from build123d import *

# Parameters (mm, degrees)
CUT_EXTRUDE_1_DEPTH = 4.5
CHAMFER_1_SIZE      = 0.5


with BuildPart() as part:
    # Эскиз1 → Повернуть1 (revolve)
    with BuildSketch(Plane.XY, mode=Mode.PRIVATE) as revolve_1_sk:
        with BuildLine():
            Line((-8, 1.5), (0, 1.5))
            Line((0, 1.5), (0, 0))
            Line((0, 0), (-9.729168699, 0))
            ThreePointArc((-9.729168699, 0), (-9.543426508, 1.350156194), (-9, 2.6))
            Line((-9, 2.6), (-8, 2.6))
            Line((-8, 2.6), (-8, 1.5))
        make_face()
    revolve(revolve_1_sk.sketch.rotate(Axis((-9.729168699, 0, 0), (1, 0, 0)), 180), axis=Axis((-9.729168699, 0, 0), (1, 0, 0)))

    # Эскиз3 → Вырез-Вытянуть1 (cut)
    with BuildSketch(Plane(origin=(-13, 0, 0), x_dir=(0, 0, -1), z_dir=(1, 0, 0))):
        Polygon((-0.25, 0.25), (-0.25, 1.5), (0.25, 1.5), (0.25, 0.25), (1.5, 0.25), (1.5, -0.25), (0.25, -0.25), (0.25, -1.5), (-0.25, -1.5), (-0.25, -0.25), (-1.5, -0.25), (-1.5, 0.25), align=None)
    extrude(amount=CUT_EXTRUDE_1_DEPTH, mode=Mode.SUBTRACT)

    # Фаска1
    chamfer_1_edges = [part.edges().sort_by_distance(p)[0] for p in [
        (0, 1.5, 0),
    ]]
    chamfer(chamfer_1_edges, length=CHAMFER_1_SIZE)


solid = part.part
The listing builds one solid part. Answer for the finished solid, in the listing's coordinates (mm). A direction names the side the tool comes from. Give positions to 0.01 mm unless a question says otherwise; leave off trailing zeros. Write each loop counter-clockwise with the first axis right and the second up, starting at its lowest first coordinate (ties: lowest second). Pieces come first, ordered by that corner, then holes.
Item 1: Which of the six approach directions +Z, -Z, +X, -X, +Y, -Y give full straight-line access (tool end or side, diameter ignored) to faces 1 (the flat face through (-8.5, 0, 0)), 2 (the cylindrical face through (-4.2, -1.43, -0.45))?
Item 2: Determine the mould class of faces 3 (the flat face through (0, 0, 0)), 4 (the cylindrical face through (-8.49, -2.48, -0.78)), 5 (the flat face through (-9, 1, 0.25)) for opening direction Y: released by +Y, released by -Y, zero draft, split by the parting line, or undercut.
Item 3: Section B-B, the plane z = 0 is taken. Write down the section's boundary in (x, y).
Item 4: Flat-ended cylindrical pins translate along their axes: P1, Ø0.6, axis at x = -9, y = -1, coming from the -Z side; P2, Ø2, axis at x = -1, y = 1.5, coming from the -Z side; P3, Ø1.3, axis at x = -9, y = -1, coming from the +Z side. Find the tip coordinate at first contact, or state that the pin passes through.
Item 5: Section D-D, the plane x = -4.25 is taken. Write down the section's boundary in (y, z), plus the area to 3 significant figures.
Item 6: Find the intervals of material crossed by line 1 along X through (y, z) = (0.1, 0.55); line 2 along X through (y, z) = (2.1, 0.55); line 3 along Y through (x, z) = (-5.75, -0.35), in increasing order.
Item 7: Section A-A, the plane x = -8.75 is taken. Write down the section's boundary in (y, z), plus the area to 3 significant figures.
Completed:
1. face 1: -X
1. face 2: +X
2. face 3: zero draft
2. face 4: split by the parting line
2. face 5: undercut
3. outline: (-9.5, -1.5) arc R5 ccw to (-9, -2.6) - (-8, -2.6) - (-8, -1.5) - (-0.5, -1.5) - (0, -1) - (0, 1) - (-0.5, 1.5) - (-8, 1.5) - (-8, 2.6) - (-9, 2.6) arc R5 ccw to (-9.5, 1.5) - (-8.5, 1.5) - (-8.5, -1.5) - close
4. P1: stops at z = -2.5
4. P2: stops at z = -1.41
4. P3: stops at z = 2.58
5. outline: circle Ø3 at (0, 0)
5. area: 7.07 mm2
6. line 1: x = -8.5 to 0
6. line 2: x = -9.23 to -8
6. line 3: y = -1.46 to 1.46
7. outline: circle Ø5.2 at (0, 0); hole (-1.5, -0.25) - (-0.25, -0.25) - (-0.25, -1.5) - (0.25, -1.5) - (0.25, -0.25) - (1.5, -0.25) - (1.5, 0.25) - (0.25, 0.25) - (0.25, 1.5) - (-0.25, 1.5) - (-0.25, 0.25) - (-1.5, 0.25) - close
7. area: 18.5 mm2
